Source: CAD feature listing. Evaluate the final solid. Frame: model axes, mm. A direction names the side the tool comes from. Give positions to 0.01 mm unless a question says otherwise; leave off trailing zeros. Loops run counter-clockwise (first coordinate to the right, second up) from the corner with the lowest first, then second, coordinate; pieces in that order, holes last. Notation, with made-up numbers: (19.5, -27) - (29.5, -27) arc R11 cw to (29.5, -12) - close; hole circle Ø4 at (-4, -14). An arc over 180 degrees is marked (long way). Write each question's results on one line, items separated by ' | '. Start each with the question number.
(1) Cut plane A-A on x = 0. Return the cut outline in (y, z).
(2) Contact query for flat-ended pins moving along their axis: pin 1 (2 mm diameter, centred on x = 5, z = 9, fed in from -Y); pin 2 (1 mm diameter, centred on y = 4.5, z = 4, fed in from -X); pin 3 (4 mm diameter, centred on y = 4, z = 6.5, fed in from +X). Output: stop coordinate, or through.
(3) Material intervals for line 1 along Z through (x, y) = (-1.5, 6); line 2 along Y through (x, z) = (0, 1.75); line 3 along X through (y, z) = (-3.75, 19), sorted ascending. Write a range as [from, to].
(4) Reachability of faces 1 (the cylindrical face through (-1.08, -4.88, 2.46)), 2 (the flat face through (2, -5, 20)), 3 (the flat face through (0, 0, 25)) from +Z, -Z, +X, -X, +Y, -Y: full face, straight path, thin tool, end or side. Return the list, or none.
(5) Cut plane C-C on z = 8.5. Return the cut outline in (x, y).
(6) Cut plane D-D on z = 20.5. Return the cut outline in (x, y).
from build123d import *

# Parameters (mm, degrees)
SKETCH_1_R      = 5
EXTRUDE_1_DEPTH = 5
SKETCH_2_R      = 7.5
EXTRUDE_2_DEPTH = 15


with BuildPart() as part:
    # 스케치1 → 보스-돌출1 (new body)
    with BuildSketch(Plane.XY):
        Circle(SKETCH_1_R)
    extrude_1 = extrude(amount=EXTRUDE_1_DEPTH)

    # 스케치2 → 보스-돌출2 (add)
    with BuildSketch(Plane.XY.offset(5)):
        Circle(SKETCH_2_R)
    extrude(amount=EXTRUDE_2_DEPTH)

    # 대칭 복사1: 보스-돌출1 across plane
    add(extrude_1.mirror(Plane(origin=(0, 0, 12.5), x_dir=(1, 0, 0), z_dir=(0, 0, -1))))


solid = part.part
Ans:
1) outline: (-7.5, 5) - (-5, 5) - (-5, 0) - (5, 0) - (5, 5) - (7.5, 5) - (7.5, 20) - (5, 20) - (5, 25) - (-5, 25) - (-5, 20) - (-7.5, 20) - close
2) pin 1: y = -6.34 | pin 2: x = -3 | pin 3: x = 7.23
3) line 1: [5, 20] | line 2: [-5, 5] | line 3: [-6.5, 6.5]
4) face 1: -Z | face 2: +Z | face 3: +Z, +X, -X, +Y, -Y
5) outline: circle Ø15 at (0, 0)
6) outline: circle Ø10 at (0, 0)
